Source: three-view drawing plus pictorial views. Frame: mm from the lowest corner of the part. Give positions to 0.01 mm unless a question says otherwise; leave off trailing zeros. Write each loop counter-clockwise with the first axis right and the second up, starting at its lowest first coordinate (ties: lowest second). Pieces come first, ordered by that corner, then holes.
Q1. Pin query (flat end, axial travel): pin 1 (4 mm diameter, centred on x = 18.5, z = 44.5, fed in from +Y); pin 2 (6 mm diameter, centred on x = 6, z = 11, fed in from -Y); pin 3 (1.5 mm diameter, centred on y = 6.5, z = 55, fed in from +X). Return the tip coordinate at first contact, or that it passes through.
Q2. Draft query along Y for the marked faces 1, 2 and 3. Return one class per face: pulls with the +Y half, pulls with the -Y half, needs draft (parallel to the pull), parting line crosses it, or undercut.
Q3. Cut plane C-C on z = 73. Return the cut outline in (x, y), plus the area to 3 significant figures.
Q4. Cut plane B-B on y = 16. Return the cut outline in (x, z).
Q5. Cut plane D-D on z = 96.35. Return the cut outline in (x, y), plus the area to 3 significant figures.
Q6. Line query: L1, parallel to Z at x = 17, y = 14.5; L2, parallel to Y at x = 23, z = 96.35; L3, parallel to Z at x = 19.5, y = 13.5. Output: solid intervals per line, ascending.
Q7. Cut plane A-A on x = 16. Return the cut outline in (y, z).
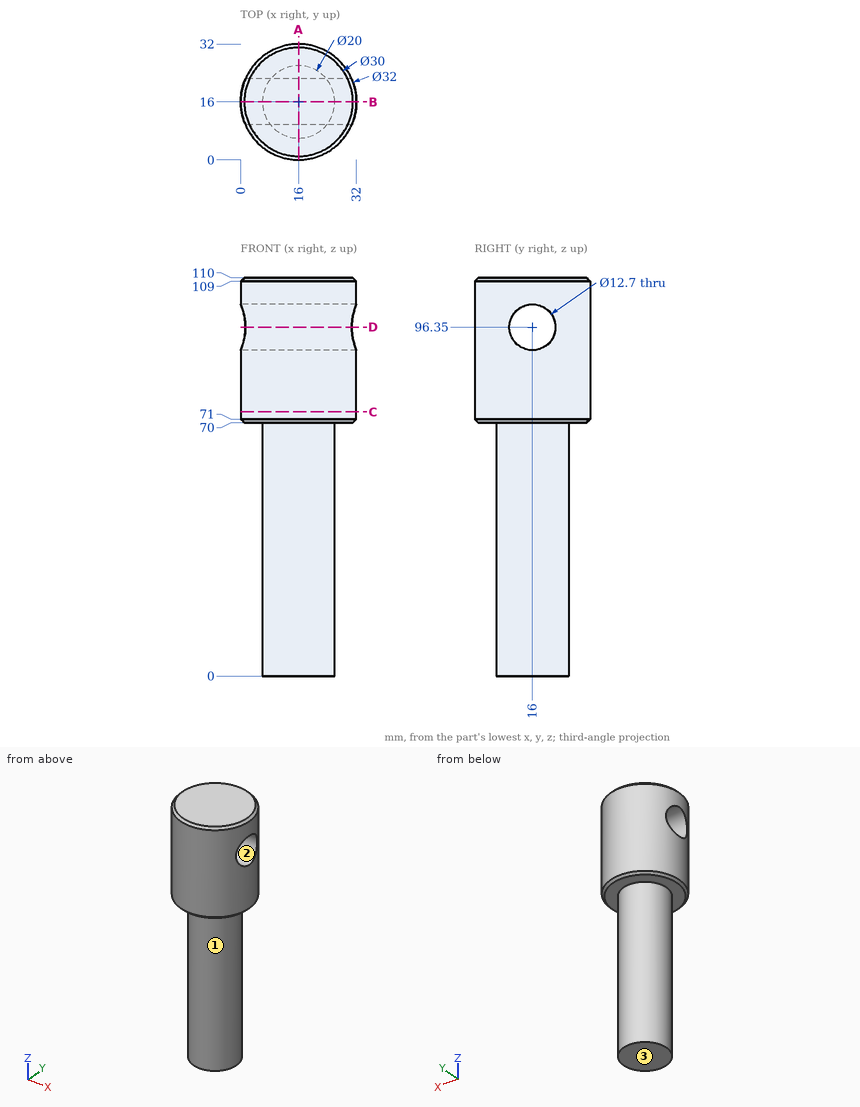
Data:
1. pin 1: stops at y = 25.99
1. pin 2: stops at y = 8.86
1. pin 3: stops at x = 20.84
2. face 1: parting line crosses it
2. face 2: undercut
2. face 3: needs draft
3. outline: circle Ø32 at (16, 16)
3. area: 804 mm2
4. outline: (0, 71) - (1, 70) - (6, 70) - (6, 0) - (26, 0) - (26, 70) - (31, 70) - (32, 71) - (32, 90) - (0, 90) - close; (0, 102.7) - (32, 102.7) - (32, 109) - (31, 110) - (1, 110) - (0, 109) - close
5. outline: (1.31, 9.65) arc R16 ccw to (30.69, 9.65) - close; (1.31, 22.35) - (30.69, 22.35) arc R16 ccw to start
5. area: 409 mm2
6. L1: z = 0 to 90.18, 102.52 to 110
6. L2: y = 1.61 to 9.65, 22.35 to 30.39
6. L3: z = 0 to 90.51, 102.19 to 110
7. outline: (0, 71) - (1, 70) - (6, 70) - (6, 0) - (26, 0) - (26, 70) - (31, 70) - (32, 71) - (32, 109) - (31, 110) - (1, 110) - (0, 109) - close; hole circle Ø12.7 at (16, 96.35)
